Check sheet for the drawn part. Datum: minimum x, y, z corner. Units: mm. A direction names the side the tool comes from. Coordinates: 2 decimals unless noted, no trailing zeros. Write each loop counter-clockwise with the first axis right and the second up, starting at its lowest first coordinate (ties: lowest second). Pieces come first, ordered by that corner, then holes. Notation, with made-up numbers: (8.5, 4.25) -> (25.5, 4.25) arc R13 cw to (25.5, 18.25) -> close; hole circle Ø7 at (51.25, 53). An arc over 180 degrees is marked (long way). Answer in a Markdown table with one row per item. Add a question column.
1. Mould release check, pull along X, two halves, no side actions. Record for the marked faces 3, 4, 5 and 6: pulls with the +X half, pulls with the -X half, needs draft (parallel to the pull), parting line crosses it, or undercut.
2. Scan lines: L1, parallel to Y at x = 78, z = 16.25; L2, parallel to X at y = 20, z = 7.75; L3, parallel to Z at x = 77.5, y = 21. Record each from-to range of solid material in increasing order. Write a range as from..to.
3. Depth check by flat-ended pin: P1, Ø8, axis at x = 95, y = 82.5, coming from the +Z side. Enter the tip coordinate at first touch or a pass-through.
4. Set-up check for the marked faces 1 and 2: record each of +Z, -Z, +X, -X, +Y, -Y from which the full face is reachable in a straight line by a thin tool's end or side.
5. Cross-section at B-B on x = 76. Record the cut outline in (y, z).
6. Cross-section at A-A on z = 22. Record the cut outline in (x, y), and give its area (3 significant figures).
7. Cross-section at C-C on y = 24. Record the cut outline in (x, z), and give its area (3 significant figures).
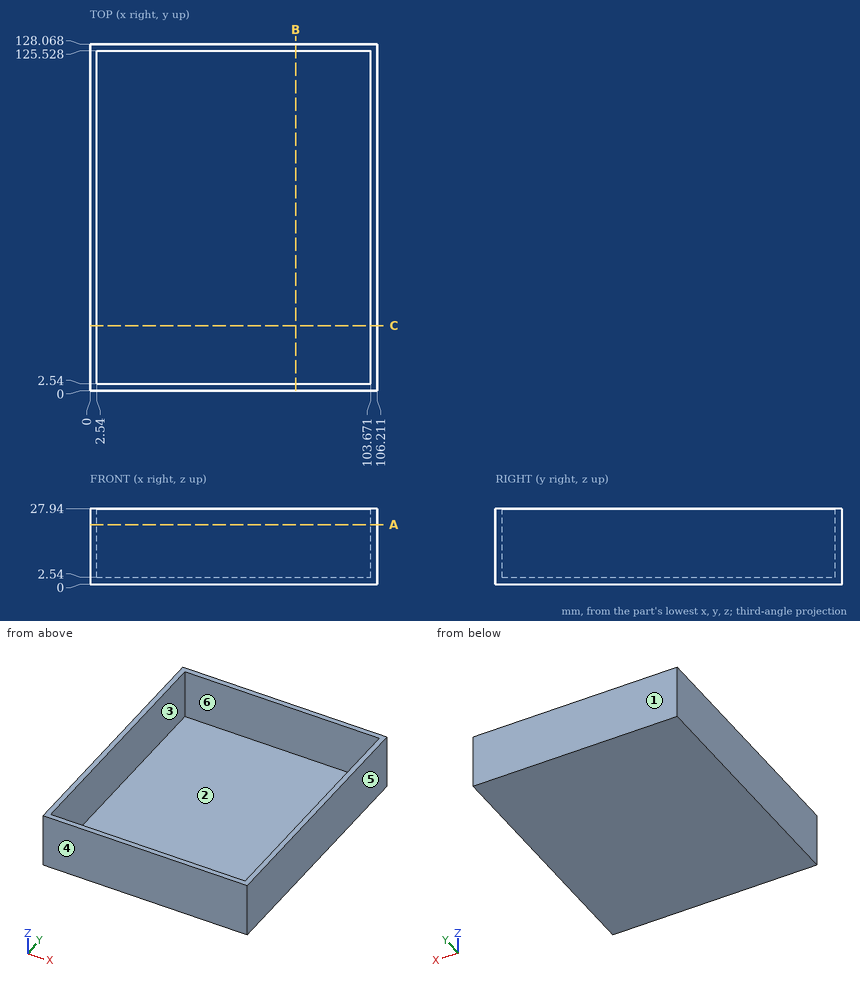
Results found:
| question | item | result |
|---|---|---|
| 1 | face 3 | undercut |
| 1 | face 4 | needs draft |
| 1 | face 5 | pulls with the +X half |
| 1 | face 6 | undercut |
| 2 | L1 | y = 0..2.54, 125.53..128.07 |
| 2 | L2 | x = 0..2.54, 103.67..106.21 |
| 2 | L3 | z = 0..2.54 |
| 3 | P1 | stops at z = 2.54 |
| 4 | face 1 | +Z, -Z, +X, -X, +Y |
| 4 | face 2 | +Z |
| 5 | outline | (0, 0) -> (128.07, 0) -> (128.07, 27.94) -> (125.53, 27.94) -> (125.53, 2.54) -> (2.54, 2.54) -> (2.54, 27.94) -> (0, 27.94) -> close |
| 6 | outline | (0, 0) -> (106.21, 0) -> (106.21, 128.07) -> (0, 128.07) -> close; hole (2.54, 2.54) -> (103.67, 2.54) -> (103.67, 125.53) -> (2.54, 125.53) -> close |
| 6 | area | 1,160 mm^2 |
| 7 | outline | (0, 0) -> (106.21, 0) -> (106.21, 27.94) -> (103.67, 27.94) -> (103.67, 2.54) -> (2.54, 2.54) -> (2.54, 27.94) -> (0, 27.94) -> close |
| 7 | area | 399 mm^2 |
